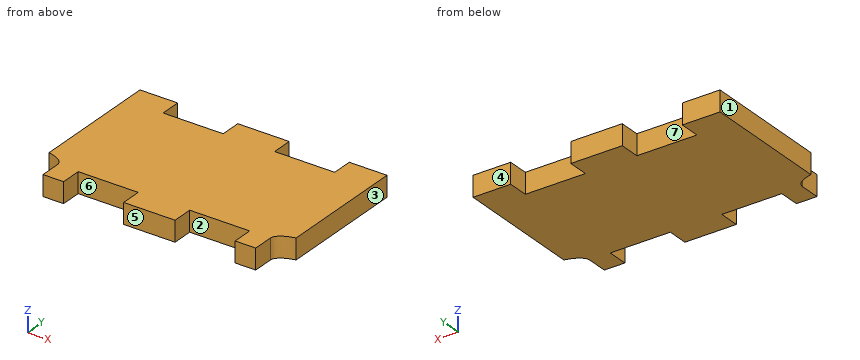
```python
from build123d import *

# Parameters (mm, degrees)
BOSS_EXTRUDE1_DEPTH = 6


with BuildPart() as part:
    # Sketch2 → Boss-Extrude1 (new body)
    with BuildSketch(Plane.XY):
        with BuildLine():
            Line((-15, 0), (-9, 0))
            Line((-9, 0), (-9, 6))
            add(Edge.make_bspline(
                [(-4, 9.583225666), (-9, 8.480694692), (-9, 6)],
                knots=[5.172942972, 5.172942972, 5.172942972, 6.283185307, 6.283185307, 6.283185307], degree=2, weights=[1, 0.849836586, 1]))
            Line((-4, 9.583225666), (-4, 41))
            Line((-4, 41), (-4, 47))
            Line((-4, 47), (-15, 47))
            Line((-15, 47), (-15, 41))
            Line((-15, 41), (-32.5, 41))
            Line((-32.5, 41), (-32.5, 47))
            Line((-32.5, 47), (-47.5, 47))
            Line((-47.5, 47), (-47.5, 41))
            Line((-47.5, 41), (-65, 41))
            Line((-65, 41), (-65, 47))
            Line((-65, 47), (-76, 47))
            Line((-76, 47), (-76, 41))
            Line((-76, 41), (-76, 9.583225666))
            add(Edge.make_bspline(
                [(-71, 6), (-71, 8.480694692), (-76, 9.583225666)],
                knots=[0, 0, 0, 1.110242335, 1.110242335, 1.110242335], degree=2, weights=[1, 0.849836586, 1]))
            Line((-71, 6), (-71, 0))
            Line((-71, 0), (-65, 0))
            Line((-65, 0), (-65, 6))
            Line((-65, 6), (-47.5, 6))
            Line((-47.5, 6), (-47.5, 0))
            Line((-47.5, 0), (-32.5, 0))
            Line((-32.5, 0), (-32.5, 6))
            Line((-32.5, 6), (-15, 6))
            Line((-15, 6), (-15, 0))
        make_face()
    extrude(amount=BOSS_EXTRUDE1_DEPTH)


solid = part.part
```
Geometry check sheet. Reference: the model listing, model coordinates, mm. Face numbers are marked on the shaded views. A direction names the side the tool comes from. Round coordinates to 2 decimals unless told otherwise and drop trailing zeros. Loops run counter-clockwise (first coordinate to the right, second up) from the corner with the lowest first, then second, coordinate; pieces in that order, holes last. Notation, with made-up numbers: (-16.75, 28.5) -> (0.25, 28.5) arc R13 cw to (0.25, 35.5) -> close; hole circle Ø11 at (-8, 47). An arc over 180 degrees is marked (long way). Use a Markdown table: item, result.
(1) Scan lines: probe 1 along X at (y, z) = (44, 1.75); probe 2 along Y at (x, z) = (-56.5, 0.75); probe 3 along Y at (x, z) = (-72, 2.75). Record each from-to range of solid material in increasing order.
Calculated:
| item | result |
|---|---|
| probe 1 | -76 to -65, -47.5 to -32.5, -15 to -4 |
| probe 2 | 6 to 41 |
| probe 3 | 7.83 to 47 |
(2) Mould release check, pull along X, two halves, no side actions. Record for the marked faces 1, 2, 3 and 4: released by +X, released by -X, zero draft, split by the parting line, or undercut.
Calculated:
| item | result |
|---|---|
| face 1 | released by -X |
| face 2 | undercut |
| face 3 | released by +X |
| face 4 | zero draft |
(3) Sectioned sample at A-A (x = -25). Enter the section's corners in (y, z).
Calculated:
| item | result |
|---|---|
| outline | (6, 0) -> (41, 0) -> (41, 6) -> (6, 6) -> close |
(4) Set-up check for the marked faces 5, 6 and 7: record each of +Z, -Z, +X, -X, +Y, -Y from which the full face is reachable in a straight line by a thin tool's end or side.
Calculated:
| item | result |
|---|---|
| face 5 | +Z, -Z, +X, -X, -Y |
| face 6 | +Z, -Z, -Y |
| face 7 | +Z, -Z, +Y |
(5) Go/stop test with flat-tipped pins: P1, Ø3, axis at x = -27.5, z = 2, coming from the +Y side; P2, Ø3, axis at y = 3, z = 2.5, coming from the +X side; P3, Ø3, axis at y = 3.5, z = 2.5, coming from the -X side. Record where each tip stops, or that it passes through.
Calculated:
| item | result |
|---|---|
| P1 | y = 41 |
| P2 | x = -9 |
| P3 | x = -71 |
